Check sheet for the modelled part. Datum: model origin and axes. Units: mm. A direction names the side the tool comes from. Round coordinates to 2 decimals unless told otherwise and drop trailing zeros. Write each loop counter-clockwise with the first axis right and the second up, starting at its lowest first coordinate (ties: lowest second). Pieces come first, ordered by that corner, then holes.
Item 1: Section check D-D, the plane z = -22. Record the cut outline in (x, y), plus the area to 3 significant figures.
Item 2: Material ranges on line 1 along Z through (x, y) = (-1.75, 1.3); line 2 along X through (y, z) = (0.45, -8.25); line 3 along X through (y, z) = (0.95, -19.25), recorded low to high.
Item 3: Section check A-A, the plane y = 0.45. Record the cut outline in (x, z), plus the area to 3 significant figures.
Item 4: Set-up check for faces 1 (the flat face through (-14, 2, -10)), 2 (the flat face through (-10, 2, -2)), 3 (the flat face through (-7.3, 0, -10.3)), 4 (the flat face through (0, 1, -11)), 5 (the flat face through (-12, 2, -15)): record each of +Z, -Z, +X, -X, +Y, -Y from which the full face is reachable in a straight line by a thin tool's end or side.
Item 5: Release check for a two-part mould opening along Z. For faces 6 (the flat face through (-7, 1, -10)), 7 (the flat face through (-10, 2, -20)), 8 (the flat face through (-12, 2, -6)) record: pulls with the +Z half, pulls with the -Z half, needs draft (parallel to the pull), parting line crosses it, or undercut.
Item 6: Depth check by flat-ended pin: pin 1 (2 mm diameter, centred on y = 3, z = -19.5, fed in from -X); pin 2 (2 mm diameter, centred on x = -12.5, y = 1.5, fed in from +Z); pin 3 (3.5 mm diameter, centred on x = -4.5, z = -14.5, fed in from -Y). Enter the tip coordinate at first touch or a pass-through.
Item 7: Section check C-C, the plane x = -4.5. Record the cut outline in (y, z).
Item 8: Section check B-B, the plane z = -16.25. Record the cut outline in (x, y), plus the area to 3 significant figures.
Autodesk Inventor part; units mm, degrees
ref_plane "YZ Plane" through (0, 0, 0) normal (1, 0, 0) x (0, 1, 0)
ref_plane "XZ Plane" through (0, 0, 0) normal (0, 1, 0) x (-1, 0, 0)
ref_plane "XY Plane" through (0, 0, 0) normal (0, 0, 1) x (1, 0, 0)
sketch "Sketch3" plane through (0, 0, 0) normal (0, 1, 0) x (-1, 0, 0)
  line L0 (0, 0) -> (7, 0)
  line L1 (7, 0) -> (7, -21)
  line L2 (7, -21) -> (0, -21)
  line L3 (0, -21) -> (0, 0)
  line L4 (10, -24) -> (10, 3)
  line L5 (10, 3) -> (-3, 3)
  line L6 (-3, 3) -> (-3, -24)
  line L7 (-3, -24) -> (10, -24)
  line L8 (10, -10.5) -> (10, -6)
  line L9 (10, -6) -> (14, -6)
  line L10 (14, -6) -> (14, -15)
  line L11 (14, -15) -> (10, -15)
  dimension "d13" = 7
  dimension "d14" = 21
  dimension "d15" = 3
  dimension "d16" = 4.5
  dimension "d17" = 4
  dimension "d18" = 9
extrude "Extrusion3" add sketch "Sketch3" along normal blind 2
sketch "Sketch4" plane through (0, 2, 0) normal (0, 1, 0) x (1, 0, 0)
  line L0 (-7, 0) -> (-7, 21)
  line L1 (-7, 21) -> (0, 21)
  line L2 (0, 21) -> (0, 0)
  line L3 (0, 0) -> (-7, 0)
  line L4 (-10, 15) -> (-14, 15)
  line L5 (-14, 15) -> (-14, 6)
  line L6 (-14, 6) -> (-10, 6)
  line L7 (-10, 6) -> (-10, -3)
  line L8 (-10, -3) -> (3, -3)
  line L9 (3, -3) -> (3, 24)
  line L10 (3, 24) -> (-10, 24)
  line L11 (-10, 24) -> (-10, 15)
extrude "Extrusion4" add sketch "Sketch4" along normal blind 2 contours L0 L1 L2 L3 | L11 L10 L9 L8 L7 L6 L5 L4
equation "\"BendRadius\" = Thickness"
equation "\"BendReliefWidth\" = Thickness"
equation "\"BendReliefDepth\" = 0.5 * Thickness"
equation "\"CornerReliefSize\" = 4 * Thickness"
equation "\"MinimumRemnant\" = 2 * Thickness"
equation "\"TransitionRadius\" = BendRadius"
equation "\"JacobiRadiusSize\" = BendRadius"
equation "\"GapSize\" = Thickness"
properties part number "basebaquela"
Values found:
1. outline: (-10, 0) - (3, 0) - (3, 4) - (-10, 4) - close
1. area: 52.0 mm2
2. line 1: z = -24 to -21, 0 to 3
2. line 2: x = -14 to -7, 0 to 3
2. line 3: x = -10 to -7, 0 to 3
3. outline: (-14, -15) - (-10, -15) - (-10, -24) - (3, -24) - (3, 3) - (-10, 3) - (-10, -6) - (-14, -6) - close; hole (-7, -21) - (0, -21) - (0, 0) - (-7, 0) - close
3. area: 240 mm2
4. face 1: +Z, -Z, -X, +Y, -Y
4. face 2: +Z, -X, +Y, -Y
4. face 3: +Z, -Z, +X, -X, -Y
4. face 4: -Y
4. face 5: -Z, -X, +Y, -Y
5. face 6: undercut
5. face 7: needs draft
5. face 8: pulls with the +Z half
6. pin 1: stops at x = -10
6. pin 2: stops at z = -6
6. pin 3: stops at y = 2
7. outline: (0, -24) - (4, -24) - (4, 3) - (0, 3) - (0, 0) - (2, 0) - (2, -21) - (0, -21) - close
8. outline: (-10, 0) - (-7, 0) - (-7, 2) - (0, 2) - (0, 0) - (3, 0) - (3, 4) - (-10, 4) - close
8. area: 38.0 mm2
